Job drawing, mm, ordinate dimensions from the low corner. One solid piece. A direction names the side the tool comes from. Give positions to 0.01 mm unless a question says otherwise; leave off trailing zeros. Loops run counter-clockwise (first coordinate to the right, second up) from the corner with the lowest first, then second, coordinate; pieces in that order, holes last.
Item 1: Probe probe 1 along Z at (x, y) = (4.75, 1.6); probe 2 along Z at (x, y) = (1.55, 3.85); probe 3 along Z at (x, y) = (5.45, 2.5). List the from-to ranges inside material, lowest first.
Item 2: Saw through at B-B on x = 3. Give the cut face in (y, z).
Item 3: Saw through at D-D on z = 2. Give the cut face in (x, y).
Item 4: Mould opens along Z. For the marked faces 1, 2, 3 and 4 say: released by +Z, released by -Z, zero draft, split by the parting line, or undercut.
Item 5: Drop flat-ended pins along their axis: P1, Ø3, axis at x = 2.5, z = 15, coming from the -Y side; P2, Ø1, axis at y = 1, z = 11.5, coming from the -X side; P3, Ø1, axis at y = 3.5, z = 3, coming from the +X side; P4, Ø3, axis at y = 2.5, z = 14.5, coming from the +X side. Give the stop position or say it passes through.
Item 6: Saw through at C-C on x = 0.8. Give the cut face in (y, z), plus the area to 3 significant figures.
Item 7: Saw through at A-A on y = 3. Give the cut face in (x, z), plus the area to 3 significant figures.
Item 8: Which spindle directions (+Z, -Z, +X, -X, +Y, -Y) get a long thin tool onto all of the face, cutting with end or side? Do the marked faces 5 and 6. Say none if no direction does.
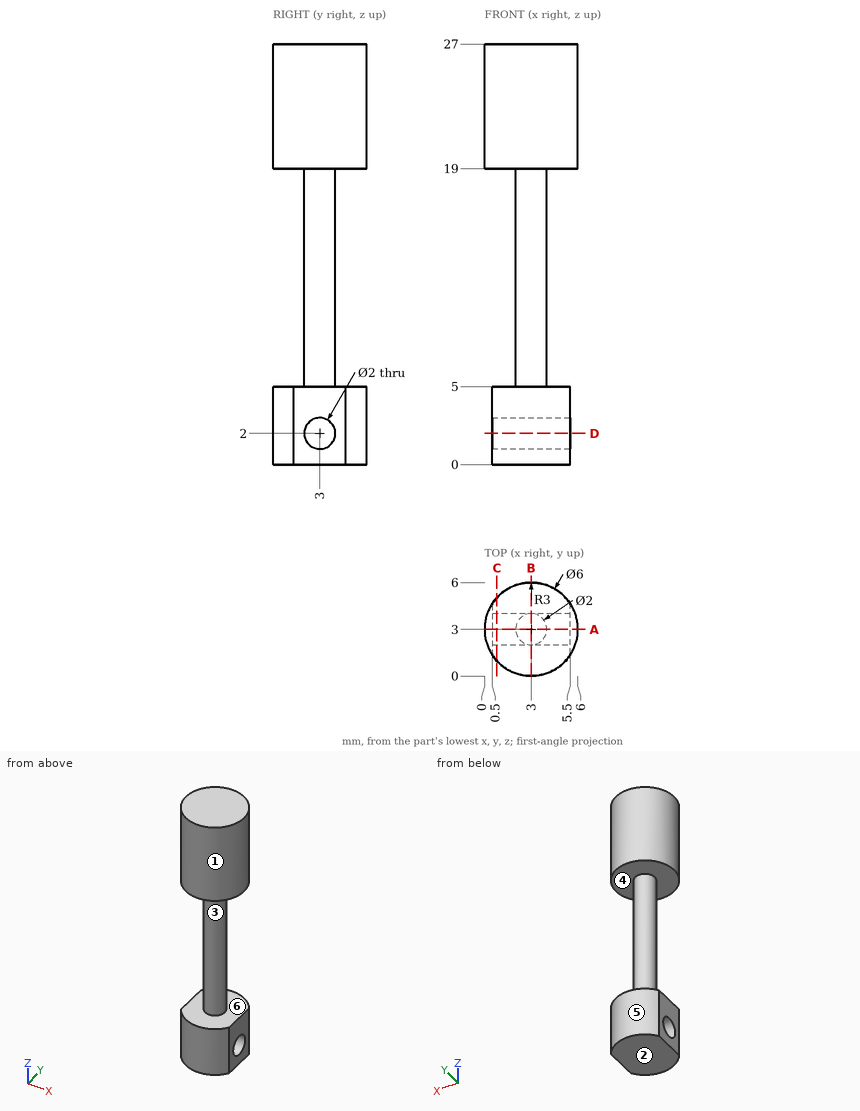
Results below:
1. probe 1: z = 0 to 5, 19 to 27
1. probe 2: z = 0 to 1.47, 2.53 to 5, 19 to 27
1. probe 3: z = 0 to 1.13, 2.87 to 5, 19 to 27
2. outline: (0, 0) - (6, 0) - (6, 5) - (4, 5) - (4, 19) - (6, 19) - (6, 27) - (0, 27) - (0, 19) - (2, 19) - (2, 5) - (0, 5) - close; hole circle Ø2 at (3, 2)
3. outline: (0.5, 1.34) arc R3 ccw to (5.5, 1.34) - (5.5, 2) - (0.5, 2) - close; (0.5, 4) - (5.5, 4) - (5.5, 4.66) arc R3 ccw to (0.5, 4.66) - close
4. face 1: zero draft
4. face 2: released by -Z
4. face 3: undercut
4. face 4: undercut
5. P1: stops at y = 2
5. P2: passes through
5. P3: stops at x = 5.5
5. P4: stops at x = 4
6. outline: (0.96, 0) - (5.04, 0) - (5.04, 5) - (0.96, 5) - close; (0.96, 19) - (5.04, 19) - (5.04, 27) - (0.96, 27) - close; hole circle Ø2 at (3, 2)
6. area: 49.9 mm2
7. outline: (0, 19) - (2, 19) - (2, 5) - (0.5, 5) - (0.5, 3) - (5.5, 3) - (5.5, 5) - (4, 5) - (4, 19) - (6, 19) - (6, 27) - (0, 27) - close; (0.5, 0) - (5.5, 0) - (5.5, 1) - (0.5, 1) - close
7. area: 91.0 mm2
8. face 5: +Z, -Z, +Y
8. face 6: none
